```python
from build123d import *

# Parameters (mm, degrees)
F1_ANGLE = 180
F3_DEPTH = 0.5
F5_DEPTH = 1.1
F5_TAPER = 10


with BuildPart() as f1:
    # F0 (on Top) → F1 (revolve)
    with BuildSketch(Plane.XY):
        with BuildLine():
            ThreePointArc((0.5062173446, 0.212), (0.9095469597, 0.517232903), (1.1512791959, 0.9615384615))
            ThreePointArc((1.1512791959, 0.9615384615), (0.6354889093, 1.358732441), (0, 1.5))
            Line((0, 1.5), (0, 0.3))
            ThreePointArc((0, 0.3), (0.2569046516, 0.2778362562), (0.5062173446, 0.212))
        make_face()
        with BuildLine():
            Line((0, -1.3), (0, -1.5))
            ThreePointArc((0, -1.5), (0.2569046516, -1.4778362562), (0.5062173446, -1.412))
            ThreePointArc((0.5062173446, -1.412), (0.2592296279, -1.3283345187), (0, -1.3))
        make_face()
        with BuildLine():
            ThreePointArc((0.5062173446, -1.412), (0.2569046516, -1.4778362562), (0, -1.5))
            Line((0, -1.5), (0, -2.7))
            ThreePointArc((0, -2.7), (0.6354889093, -2.558732441), (1.1512791959, -2.1615384615))
            ThreePointArc((1.1512791959, -2.1615384615), (0.9095469597, -1.717232903), (0.5062173446, -1.412))
        make_face()
        with BuildLine():
            ThreePointArc((0, 1.5), (0.6354889093, 1.358732441), (1.1512791959, 0.9615384615))
            ThreePointArc((1.1512791959, 0.9615384615), (1.1328359299, 1.6958317266), (0.6899514895, 2.2818181818))
            ThreePointArc((0.6899514895, 2.2818181818), (0.4512608599, 1.864870449), (0, 1.7))
            Line((0, 1.7), (0, 1.5))
        make_face()
        with BuildLine():
            ThreePointArc((0.5062173446, 0.212), (1.0243861064, -0.1042659515), (1.3747727085, -0.6))
            ThreePointArc((1.3747727085, -0.6), (1.4848687308, 0.2125202398), (1.1512791959, 0.9615384615))
            ThreePointArc((1.1512791959, 0.9615384615), (0.9095469597, 0.517232903), (0.5062173446, 0.212))
        make_face()
        with BuildLine():
            ThreePointArc((0, -1.3), (0.2592296279, -1.3283345187), (0.5062173446, -1.412))
            ThreePointArc((0.5062173446, -1.412), (1.0243861064, -1.0957340485), (1.3747727085, -0.6))
            ThreePointArc((1.3747727085, -0.6), (1.0243861064, -0.1042659515), (0.5062173446, 0.212))
            ThreePointArc((0.5062173446, 0.212), (0.2592296279, 0.1283345187), (0, 0.1))
            Line((0, 0.1), (0, -1.3))
        make_face()
        with BuildLine():
            ThreePointArc((1.3747727085, -0.6), (1.0243861064, -1.0957340485), (0.5062173446, -1.412))
            ThreePointArc((0.5062173446, -1.412), (0.9095469597, -1.717232903), (1.1512791959, -2.1615384615))
            ThreePointArc((1.1512791959, -2.1615384615), (1.4848687308, -1.4125202398), (1.3747727085, -0.6))
        make_face()
        with BuildLine():
            ThreePointArc((1.1512791959, -2.1615384615), (0.6354889093, -2.558732441), (0, -2.7))
            Line((0, -2.7), (0, -2.9))
            ThreePointArc((0, -2.9), (0.4512608599, -3.064870449), (0.6899514895, -3.4818181818))
            ThreePointArc((0.6899514895, -3.4818181818), (1.1328359299, -2.8958317266), (1.1512791959, -2.1615384615))
        make_face()
        with BuildLine():
            Line((0, 0.3), (0, 0.1))
            ThreePointArc((0, 0.1), (0.2592296279, 0.1283345187), (0.5062173446, 0.212))
            ThreePointArc((0.5062173446, 0.212), (0.2569046516, 0.2778362562), (0, 0.3))
        make_face()
        with BuildLine():
            ThreePointArc((0, 2.5), (0.3618136135, 2.4441551071), (0.6899514895, 2.2818181818))
            ThreePointArc((0.6899514895, 2.2818181818), (0.535129551, 2.8512608599), (0, 3.1))
            Line((0, 3.1), (0, 2.5))
        make_face()
        with BuildLine():
            ThreePointArc((0, 1.7), (0.4512608599, 1.864870449), (0.6899514895, 2.2818181818))
            ThreePointArc((0.6899514895, 2.2818181818), (0.3618136135, 2.4441551071), (0, 2.5))
            Line((0, 2.5), (0, 1.7))
        make_face()
        with BuildLine():
            ThreePointArc((0, -4.3), (0.535129551, -4.0512608599), (0.6899514895, -3.4818181818))
            ThreePointArc((0.6899514895, -3.4818181818), (0.3618136135, -3.6441551071), (0, -3.7))
            Line((0, -3.7), (0, -4.3))
        make_face()
        with BuildLine():
            ThreePointArc((0.6899514895, -3.4818181818), (0.4512608599, -3.064870449), (0, -2.9))
            Line((0, -2.9), (0, -3.7))
            ThreePointArc((0, -3.7), (0.3618136135, -3.6441551071), (0.6899514895, -3.4818181818))
        make_face()
    revolve(axis=Axis((0, -0.6, 0), (0, -1, 0)), revolution_arc=F1_ANGLE)

    # F2 (on face) → F3 (join)
    with BuildSketch(Plane(origin=(0, 0, 0), x_dir=(1, 0, 0), z_dir=(0, 0, -1))):
        with BuildLine():
            ThreePointArc((-1.3747727085, 0.6), (-1.4848687308, -0.2125202398), (-1.1512791959, -0.9615384615))
            ThreePointArc((-1.1512791959, -0.9615384615), (-1.1328359299, -1.6958317266), (-0.6899514895, -2.2818181818))
            ThreePointArc((-0.6899514895, -2.2818181818), (-0.535129551, -2.8512608599), (0, -3.1))
            ThreePointArc((0, -3.1), (0.535129551, -2.8512608599), (0.6899514895, -2.2818181818))
            ThreePointArc((0.6899514895, -2.2818181818), (1.1328359299, -1.6958317266), (1.1512791959, -0.9615384615))
            ThreePointArc((1.1512791959, -0.9615384615), (1.4848687308, -0.2125202398), (1.3747727085, 0.6))
            ThreePointArc((1.3747727085, 0.6), (1.4848687308, 1.4125202398), (1.1512791959, 2.1615384615))
            ThreePointArc((1.1512791959, 2.1615384615), (1.1328359299, 2.8958317266), (0.6899514895, 3.4818181818))
            ThreePointArc((0.6899514895, 3.4818181818), (0.535129551, 4.0512608599), (0, 4.3))
            ThreePointArc((0, 4.3), (-0.535129551, 4.0512608599), (-0.6899514895, 3.4818181818))
            ThreePointArc((-0.6899514895, 3.4818181818), (-1.1328359299, 2.8958317266), (-1.1512791959, 2.1615384615))
            ThreePointArc((-1.1512791959, 2.1615384615), (-1.4848687308, 1.4125202398), (-1.3747727085, 0.6))
        make_face()
    extrude(amount=F3_DEPTH)

    # F4 (on face) → F5 (cut)
    with BuildSketch(Plane(origin=(0, 0, -0.5), x_dir=(1, 0, 0), z_dir=(0, 0, -1))):
        with BuildLine():
            ThreePointArc((0.4, 4.1744562647), (0, 4.3), (-0.4, 4.1744562647))
            Line((-0.4, 4.1744562647), (-0.4, -2.9744562647))
            ThreePointArc((-0.4, -2.9744562647), (0, -3.1), (0.4, -2.9744562647))
            Line((0.4, -2.9744562647), (0.4, 4.1744562647))
        make_face()
        with BuildLine():
            ThreePointArc((0.4, -2.9744562647), (0, -3.1), (-0.4, -2.9744562647))
            Line((-0.4, -2.9744562647), (-0.4, -6.0718938156))
            Line((-0.4, -6.0718938156), (0.4, -6.0718938156))
            Line((0.4, -6.0718938156), (0.4, -2.9744562647))
        make_face()
        with BuildLine():
            Line((0.4, 6.0718938156), (-0.4, 6.0718938156))
            Line((-0.4, 6.0718938156), (-0.4, 4.1744562647))
            ThreePointArc((-0.4, 4.1744562647), (0, 4.3), (0.4, 4.1744562647))
            Line((0.4, 4.1744562647), (0.4, 6.0718938156))
        make_face()
    extrude(amount=-F5_DEPTH, taper=F5_TAPER, mode=Mode.SUBTRACT)


solid = f1.part
```
Can you work these out from the model? Positions are in its coordinate system, mm. Coordinates: 2 decimals unless noted, no trailing zeros. Loops run counter-clockwise (first coordinate to the right, second up) from the corner with the lowest first, then second, coordinate; pieces in that order, holes last.
1) Imagine slicing it at B-B on z = 1. List the corners of the cut face in (x, y) for me.
2) Imagine slicing it at C-C on z = 1.3. List the corners of the cut face in (x, y) for me, plus the area to 3 significant figures.
3) I need wall thicknesses on probe 1 along X at (y, z) = (1.5, 0.3); probe 2 along Z at (x, y) = (-0.9, -1.25); probe 3 along X at (y, z) = (-3, 0.5). Which ranges of each line are inside material? Lowest first, please.
4) Imagine slicing it at A-A on x = 0.5. List the corners of the cut face in (y, z) for me.
Completed:
1. outline: (-0.94, -0.6) arc R1.12 ccw to (-0.57, -2.16) arc R0.66 ccw (long way) to (0.57, -2.16) arc R1.12 ccw to (0.94, -0.6) arc R1.12 ccw to (0.57, 0.96) arc R0.66 ccw (long way) to (-0.57, 0.96) arc R1.12 ccw to start
2. outline: (-0.45, -0.6) arc R0.75 ccw (long way) to (0.45, -0.6) arc R0.75 ccw (long way) to start
2. area: 3.34 mm2
3. probe 1: x = -1.14 to -0.26, 0.26 to 1.14
3. probe 2: z = -0.5 to 1.2
3. probe 3: x = -0.97 to -0.22, 0.22 to 0.97
4. outline: (-4.09, -0.5) - (2.89, -0.5) - (2.89, 0) arc R0.49 ccw to (2.28, 0.48) arc R1.09 ccw to (0.96, 1.04) arc R1.41 ccw to (-0.6, 1.28) arc R1.41 ccw to (-2.16, 1.04) arc R1.09 ccw to (-3.48, 0.48) arc R0.49 ccw to (-4.09, 0) - close
